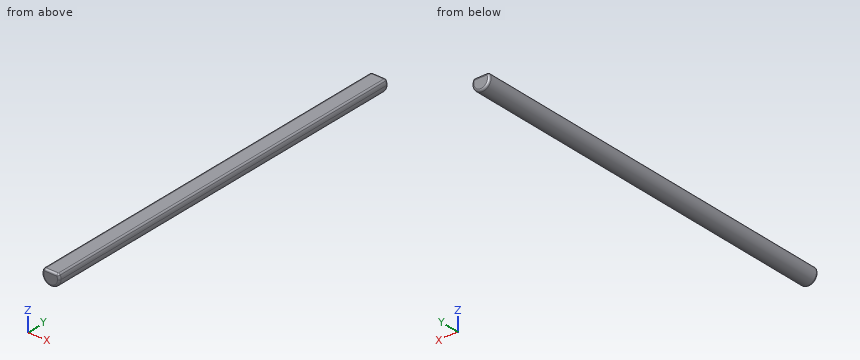
from build123d import *

# Parameters (mm, degrees)
F1_DEPTH = 101.6
F2_R     = 0.508


with BuildPart() as f1:
    # F0 (on Front) → F1 (new body)
    with BuildSketch(Plane.XZ):
        with BuildLine():
            ThreePointArc((-1.9007619525, 1.27), (-0.6635714644, -2.1875714644), (2.286, 0))
            ThreePointArc((2.286, 0), (2.1875714644, 0.6635714644), (1.9007619525, 1.27))
            Line((1.9007619525, 1.27), (-1.9007619525, 1.27))
        make_face()
    extrude(amount=F1_DEPTH)

    # F2
    f2_edges = [f1.edges().sort_by_distance(p)[0] for p in [
        (-1.900762, -50.8, 1.27),
        (0, -101.6, 1.27),
        (-0.663571, -101.6, -2.187571),
        (0, 0, 1.27),
        (-0.663571, 0, -2.187571),
        (1.900762, -50.8, 1.27),
    ]]
    fillet(f2_edges, radius=F2_R)


solid = f1.part
For this review, take the finished solid that the model builds, in its own axes (mm). Give positions to 0.01 mm unless a question says otherwise; leave off trailing zeros. Order: outer loops, then holes, each group sorted by start corner. A loop starts at its lowest first (then second) coordinate and runs counter-clockwise, first axis right, second up. Notation, with made-up numbers: (-14, 58) -> (1, 58) arc R9 cw to (1, 73) -> close; hole circle Ø11 at (69.25, 78.5). An arc over 180 degrees is marked (long way). Write item = value, one per line.
1) Insertion check: pin 1 (1.5 mm diameter, centred on x = -0.5, z = 0, fed in from +Y); pin 2 (2 mm diameter, centred on x = -1.5, y = -57.5, fed in from -Z). Each pin has a flat end and moves straight along its axis. Give the tip position at first contact, or say it passes through.
Findings:
pin_1 = 0
pin_2 = -2.23
2) We need section A-A, the plane y = -64. Give the boundary of the cut face in (x, z), and give its area (3 significant figures).
Findings:
outline = (-2.07, 0.98) arc R2.29 ccw (long way) to (2.07, 0.98) arc R0.51 ccw to (1.61, 1.27) -> (-1.61, 1.27) arc R0.51 ccw to start
area = 13.7 mm^2
3) To check wall thickness, follow L1, parallel to X at y = -59, z = 0.2; L2, parallel to Z at x = -0.1, y = -79.5; L3, parallel to X at y = -83.5, z = -2. State the ranges of each line that lie inside material, in increasing order. Write a range as from..to.
Findings:
L1 = -2.28..2.28
L2 = -2.28..1.27
L3 = -1.11..1.11
